Job drawing, mm, ordinate dimensions from the low corner. One solid piece. A direction names the side the tool comes from. Round coordinates to 2 decimals unless told otherwise and drop trailing zeros. Write each loop counter-clockwise with the first axis right and the second up, starting at its lowest first coordinate (ties: lowest second). Pieces come first, ordered by that corner, then holes. Notation, with made-up numbers: M -6,16 L 20,16 A23 cw 20,27 Z; hole C -0.5,-20 d11. An arc over 180 degrees is marked long. Write each question's results on one line, items separated by ' | '. Start each with the question number.
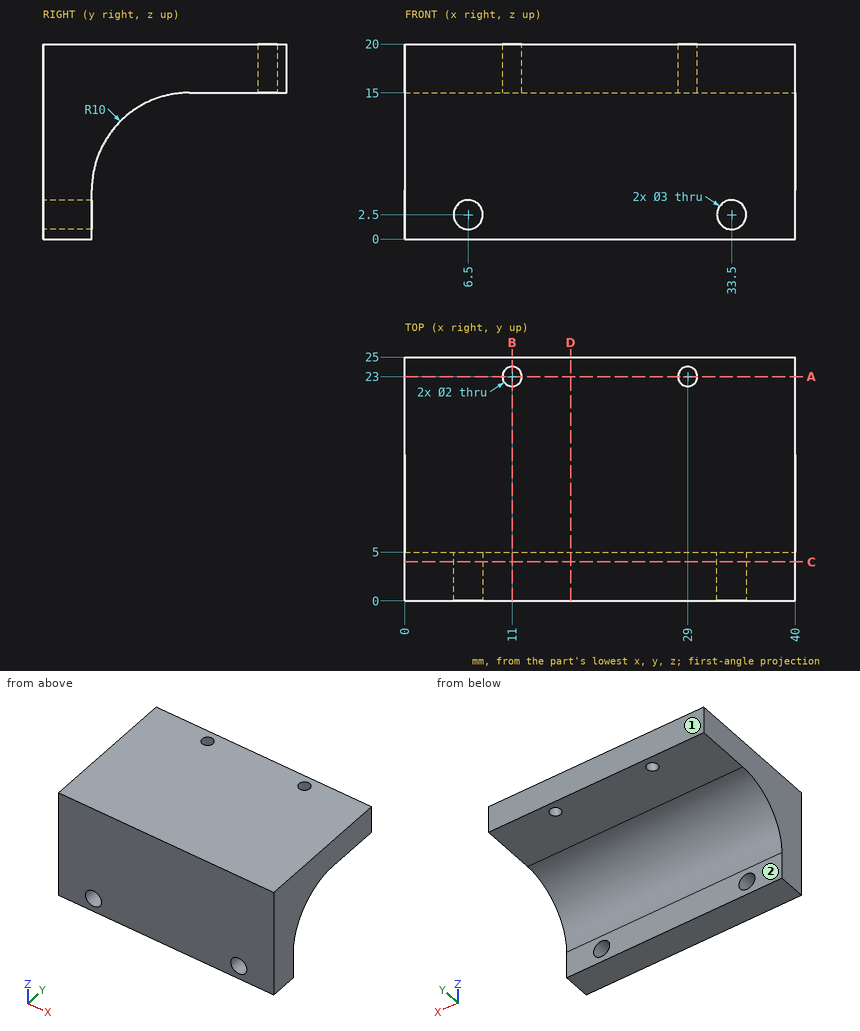
1) Saw through at B-B, the plane x = 11. Write the cut outline in (y, z).
2) Saw through at A-A, the plane y = 23. Write the cut outline in (x, z).
3) Saw through at C-C, the plane y = 4. Write the cut outline in (x, z), plus the area to 3 significant figures.
4) Drop flat-ended pins along their axis: pin 1 Ø8 at (x, z) = (6.5, 5) entering from +Y; pin 2 Ø3 at (x, y) = (16.5, 18) entering from -Z; pin 3 Ø12 at (x, z) = (22, 16.5) entering from -Y; pin 4 Ø1.6 at (x, y) = (11, 23) entering from -Z. Give the stop position or say it passes through.
5) 3-axis set-ups, long thin cutter, end or side, ignore diameter. For the marked faces 1 and 2: which of +Z, -Z, +X, -X, +Y, -Y reach the whole face in a straight line?
6) Wall check: line 1 along X through (y, z) = (1.75, 2.5); line 2 along Z through (x, y) = (6.5, 3.75); line 3 along Z through (x, y) = (5, 21). Give the ranges that are in metal, low to high. Write a range as from..to.
7) Saw through at D-D, the plane x = 17. Write the cut outline in (y, z).
Filled sheet:
1) outline: M 0,0 L 5,0 L 5,5 A10 cw 15,15 L 22,15 L 22,20 L 0,20 Z; M 24,15 L 25,15 L 25,20 L 24,20 Z
2) outline: M 0,15 L 10,15 L 10,20 L 0,20 Z; M 12,15 L 28,15 L 28,20 L 12,20 Z; M 30,15 L 40,15 L 40,20 L 30,20 Z
3) outline: M 0,0 L 40,0 L 40,20 L 0,20 Z; hole C 6.5,2.5 d3; hole C 33.5,2.5 d3 | area: 786 mm^2
4) pin 1: stops at y = 5.83 | pin 2: stops at z = 15 | pin 3: stops at y = 0 | pin 4: passes through
5) face 1: +Z, -Z, +X, -X, +Y | face 2: -Z, +X, -X, +Y
6) line 1: x = 0..5, 8..32, 35..40 | line 2: z = 0..1, 4..20 | line 3: z = 15..20
7) outline: M 0,0 L 5,0 L 5,5 A10 cw 15,15 L 25,15 L 25,20 L 0,20 Z
